For this review, use the dimensioned drawing (mm, ordinates from the lowest corner) and the shaded views. A direction names the side the tool comes from. Give positions to 0.01 mm unless a question says otherwise; leave off trailing zeros. Write each loop counter-clockwise with the first axis right and the second up, starting at its lowest first coordinate (ties: lowest second). Pieces come first, ordered by that corner, then holes. Notation, with made-up numbers: (0, 64) -> (6, 64) arc R31 cw to (6, 103) -> close; hole circle Ø3 at (-4, 37.5). An arc over 180 degrees is marked (long way). Answer as CSV lines item,"result".
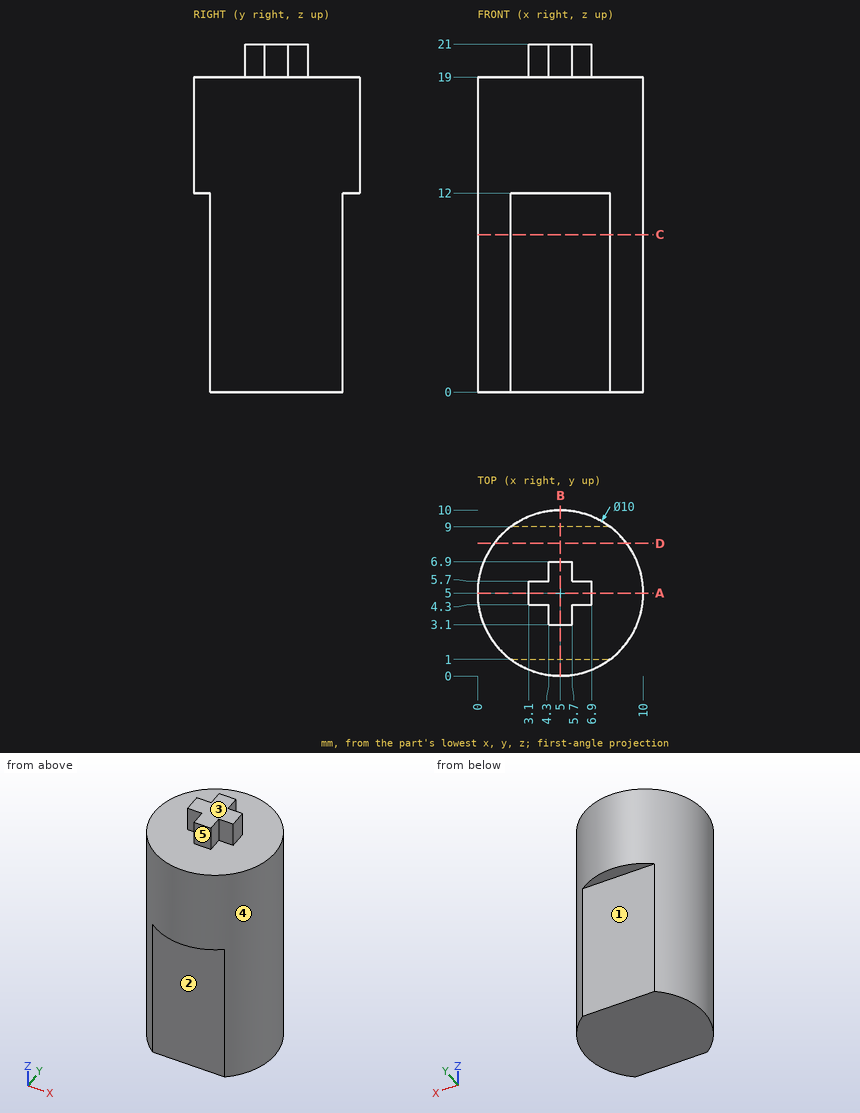
Q1. Clearance check with flat-ended pins moving along their axes: pin 1 (5 mm diameter, centred on x = 2, z = 4, fed in from +Y); pin 2 (1.5 mm diameter, centred on x = 3.5, z = 15, fed in from +Y); pin 3 (5 mm diameter, centred on x = 3.5, z = 8, fed in from -Y). State where each tip first meets the part, or that it passes through.
Answer block:
pin 1,"stops at y = 9"
pin 2,"stops at y = 9.94"
pin 3,"stops at y = 1"
Q2. Add section C-C (z = 9.5). Write out the cut boundary in (x, y).
Answer block:
outline,"(2, 1) -> (8, 1) arc R5 ccw to (8, 9) -> (2, 9) arc R5 ccw to start"
Q3. Add section D-D (y = 8). Write out the cut boundary in (x, z), plus the area to 3 significant figures.
Answer block:
outline,"(1, 0) -> (9, 0) -> (9, 19) -> (1, 19) -> close"
area,"152 mm2"
Q4. Add section B-B (x = 5). Write out the cut boundary in (y, z).
Answer block:
outline,"(0, 12) -> (1, 12) -> (1, 0) -> (9, 0) -> (9, 12) -> (10, 12) -> (10, 19) -> (6.9, 19) -> (6.9, 21) -> (3.1, 21) -> (3.1, 19) -> (0, 19) -> close"
Q5. For the marked faces 1, 2, 3, 4 and 5, list the 3-axis set-ups (+Z, -Z, +X, -X, +Y, -Y) from which the entire face can be reached by the end or side of a thin tool; tool diameter is ignored.
Answer block:
face 1,"-Z, +X, -X, +Y"
face 2,"-Z, +X, -X, -Y"
face 3,"+Z, +X, -X, +Y, -Y"
face 4,"+Z, -Z"
face 5,"+Z, +X, -X, -Y"
Q6. To check wall thickness, follow probe 1 along Y at (x, z) = (6.5, 7.5); probe 2 along Z at (x, y) = (5.25, 8); probe 3 along Z at (x, y) = (4, 9.5). State the ranges of each line that lie inside material, in increasing order. Write a range as [from, to].
Answer block:
probe 1,"y = [1, 9]"
probe 2,"z = [0, 19]"
probe 3,"z = [12, 19]"
Q7. Add section A-A (y = 5). Write out the cut boundary in (x, z), plus the area to 3 significant figures.
Answer block:
outline,"(0, 0) -> (10, 0) -> (10, 19) -> (6.9, 19) -> (6.9, 21) -> (3.1, 21) -> (3.1, 19) -> (0, 19) -> close"
area,"198 mm2"
